Verification items for the finished model (mm, model axes). A direction names the side the tool comes from. Round coordinates to 2 decimals unless told otherwise and drop trailing zeros. One line per item, written item: value.
from build123d import *

# Parameters (mm, degrees)
SKETCH2_W           = 1219.2
SKETCH2_H           = 38.1
BOSS_EXTRUDE2_DEPTH = 19.05
SKETCH3_R           = 3.175
CUT_EXTRUDE1_DEPTH  = 19.05
CUT_EXTRUDE2_DEPTH  = 9.525


with BuildPart() as part:
    # Sketch2 → Boss-Extrude2 (new body)
    with BuildSketch(Plane(origin=(0, 0, 0), x_dir=(1, 0, 0), z_dir=(0, 1, 0))):
        with Locations((-609.6, -19.05)):
            Rectangle(SKETCH2_W, SKETCH2_H)
    extrude(amount=BOSS_EXTRUDE2_DEPTH)

    # Sketch3 → Cut-Extrude1 (cut)
    with BuildSketch(Plane(origin=(0, 19.05, 0), x_dir=(1, 0, 0), z_dir=(0, 1, 0))):
        with Locations(Location((-19.05, -19.05, 0), (0, 0, 270))):
            Circle(SKETCH3_R)
        with Locations(Location((-323.85, -19.05, 0), (0, 0, 270))):
            Circle(SKETCH3_R)
    extrude(amount=-CUT_EXTRUDE1_DEPTH, mode=Mode.SUBTRACT)

    # Sketch4 → Cut-Extrude2 (cut)
    with BuildSketch(Plane(origin=(0, 19.05, 0), x_dir=(1, 0, 0), z_dir=(0, 1, 0))):
        with BuildLine():
            Line((-316.143895572, 0), (-322.659375, -16.106696225))
            ThreePointArc((-322.659375, -16.106696225), (-321.217429073, -17.275121043), (-320.675, -19.05))
            ThreePointArc((-320.675, -19.05), (-320.733462299, -19.656479808), (-320.906696225, -20.240625))
            Line((-320.906696225, -20.240625), (-306.190177353, -26.19375))
            Line((-306.190177353, -26.19375), (-295.594283764, 0))
            Line((-295.594283764, 0), (-316.143895572, 0))
        make_face()
        with BuildLine():
            ThreePointArc((-326.793303775, -17.859375), (-325.089331047, -16.126870931), (-322.659375, -16.106696225))
            Line((-322.659375, -16.106696225), (-316.143895572, 0))
            Line((-316.143895572, 0), (-336.69350738, 0))
            Line((-336.69350738, 0), (-341.509822647, -11.90625))
            Line((-341.509822647, -11.90625), (-326.793303775, -17.859375))
        make_face()
        with BuildLine():
            ThreePointArc((-320.906696225, -20.240625), (-325.040625, -21.993303775), (-326.793303775, -17.859375))
            Line((-326.793303775, -17.859375), (-341.509822647, -11.90625))
            Line((-341.509822647, -11.90625), (-348.653572647, -29.566072647))
            Line((-348.653572647, -29.566072647), (-327.557139607, -38.1))
            Line((-327.557139607, -38.1), (-311.00649262, -38.1))
            Line((-311.00649262, -38.1), (-306.190177353, -26.19375))
            Line((-306.190177353, -26.19375), (-320.906696225, -20.240625))
        make_face()
        with BuildLine():
            Line((-35.448406744, -28.745089286), (-29.917583168, -38.1))
            Line((-29.917583168, -38.1), (-13.839851848, -38.1))
            Line((-13.839851848, -38.1), (0, -29.917583168))
            Line((0, -29.917583168), (0, -13.839851848))
            Line((0, -13.839851848), (-2.651593256, -9.354910714))
            Line((-2.651593256, -9.354910714), (-16.316932209, -17.434151786))
            ThreePointArc((-16.316932209, -17.434151786), (-15.987475287, -18.212403807), (-15.875, -19.05))
            ThreePointArc((-15.875, -19.05), (-18.212403807, -22.112524713), (-21.783067791, -20.665848214))
            Line((-21.783067791, -20.665848214), (-35.448406744, -28.745089286))
        make_face()
        with BuildLine():
            Line((-30.31276801, 0), (-52.443119188, 0))
            Line((-52.443119188, 0), (-35.448406744, -28.745089286))
            Line((-35.448406744, -28.745089286), (-21.783067791, -20.665848214))
            ThreePointArc((-21.783067791, -20.665848214), (-22.125147998, -18.260006461), (-20.665848214, -16.316932209))
            Line((-20.665848214, -16.316932209), (-30.31276801, 0))
        make_face()
        with BuildLine():
            Line((-8.182416832, 0), (-30.31276801, 0))
            Line((-30.31276801, 0), (-20.665848214, -16.316932209))
            ThreePointArc((-20.665848214, -16.316932209), (-18.260006461, -15.974852002), (-16.316932209, -17.434151786))
            Line((-16.316932209, -17.434151786), (-2.651593256, -9.354910714))
            Line((-2.651593256, -9.354910714), (-8.182416832, 0))
        make_face()
    extrude(amount=-CUT_EXTRUDE2_DEPTH, mode=Mode.SUBTRACT)


solid = part.part
(1) Depth check by flat-ended pin: pin 1 Ø11.5 at (x, z) = (-30.5, 10.5) entering from +Y (3 decimals); pin 2 Ø4 at (x, z) = (-19.05, 19.05) entering from +Y; pin 3 Ø1.5 at (y, z) = (12, 16) entering from +X. Enter the tip coordinate at first touch or a pass-through.
Completed:
pin 1: stops at y = 9.525
pin 2: passes through
pin 3: stops at x = -42.54
(2) Mould release check, pull along X, two halves, no side actions. Record for faces 1 (the face through (-1219.2, 9, 19)), 2 (the face through (-780, 19.05, 19)), 3 (the face through (-21, 9.525, 15)): +X half, -X half, draft (parallel to the pull), parting line (faces both ways), or undercut.
Completed:
face 1: -X half
face 2: draft
face 3: undercut
(3) Thickness scan on L1, parallel to X at y = 6.25, z = 19.05 (3 decimals); L2, parallel to Z at x = -19.05, y = 3 (3 decimals); L3, parallel to X at y = 11, z = 8.5. Record the ranges inside material, lowest first. Write a range as from..to.
Completed:
L1: x = -1219.2..-327.025, -320.675..-22.225, -15.875..0
L2: z = 0..15.875, 22.225..38.1
L3: x = -1219.2..-340.13, -299.03..-47.42, -3.16..0
(4) Tool access check on faces 4 (the face through (-618, 9, 0)), 5 (the face through (-322, 9.525, 15)). Record the directions out of +Z, -Z, +X, -X, +Y, -Y that give a thin tool (end or side, any length) a straight path to the whole face; none if there is none.
Completed:
face 4: -Z, +X, -X, +Y, -Y
face 5: +Y
